The model under review builds one solid part; all positions refer to its coordinate system, in mm. A direction names the side the tool comes from. Coordinates: 2 decimals unless noted, no trailing zeros. Loops run counter-clockwise (first coordinate to the right, second up) from the corner with the lowest first, then second, coordinate; pieces in that order, holes last. Notation, with made-up numbers: M 39.5,82.25 L 69.5,82.25 A9 cw 69.5,94.25 Z; hole C 11,6.5 d8. An arc over 180 degrees is marked long. Use one line per item in the form item = value.
```python
from build123d import *

# Parameters (mm, degrees)
F0_W     = 30
F0_H     = 40
F0_W_2   = 20
F0_H_2   = 8
F2_DEPTH = 3
F1_W     = 20
F1_H     = 3
F3_DEPTH = 1
F4_R     = 0.5


with BuildPart() as f2:
    # F0 (on Top) → F2 (new body)
    with BuildSketch(Plane.XY):
        Rectangle(F0_W, F0_H)
        with Locations((0, 11.941392)):
            Rectangle(F0_W_2, F0_H_2, mode=Mode.SUBTRACT)
    extrude(amount=F2_DEPTH)

    # F1 (on face) → F3 (join)
    with BuildSketch(Plane.XY):
        with Locations((0, 15.365714)):
            Rectangle(F1_W, F1_H)
    extrude(amount=F3_DEPTH)

    # F4
    f4_edges = [f2.edges().sort_by_distance(p)[0] for p in [
        (15, 0, 0),
        (0, 20, 0),
        (-15, 0, 0),
        (0, -20, 0),
        (-15, -20, 1.5),
        (15, -20, 1.5),
        (-15, 20, 1.5),
        (15, 20, 1.5),
    ]]
    fillet(f4_edges, radius=F4_R)


solid = f2.part
```
1. Wall thickness on line 1 along X through (y, z) = (11, 0.65); line 2 along Y through (x, z) = (2.5, 2.5); line 3 along Y through (x, z) = (-3, 0.95): over which ranges is each line inside the solid? List them lowest first. Write a range as from..to.
Response values:
line_1 = -15..-10, 10..15
line_2 = -20..7.94, 15.94..20
line_3 = -20..7.94, 13.87..20
2. Insertion check: P1, Ø8, axis at x = 1.5, y = 9, coming from the -Z side; P2, Ø0.6, axis at x = -4.5, y = 15, coming from the +Z side. Each pin has a flat end and moves straight along its axis. Give the tip position at first contact, or say it passes through.
Response values:
P1 = 0
P2 = 1
3. Add section C-C (y = 13). State the section outline as (x, z) points.
Response values:
outline = M -15,0.5 A0.5 ccw -14.5,0 L -10,0 L -10,3 L -15,3 Z; M 10,0 L 14.5,0 A0.5 ccw 15,0.5 L 15,3 L 10,3 Z
4. Add section B-B (z = 2.05). State the section outline as (x, y) points.
Response values:
outline = M -15,-19.5 A0.5 ccw -14.5,-20 L 14.5,-20 A0.5 ccw 15,-19.5 L 15,19.5 A0.5 ccw 14.5,20 L -14.5,20 A0.5 ccw -15,19.5 Z; hole M -10,7.94 L 10,7.94 L 10,15.94 L -10,15.94 Z
5. The part is to be moulded in two halves that separate along Y. For faces 4 (the face through (-15, 0, 2)), 5 (the face through (-0.1, 13.866, 0.5)), 6 (the face through (0, -20, 2)), say which applies: pulls with the +Y half, pulls with the -Y half, needs draft (parallel to the pull), parting line crosses it, or undercut.
Response values:
face_4 = needs draft
face_5 = undercut
face_6 = pulls with the -Y half
6. Machinability: for faces 1 (the face through (0, 20, 2)), 2 (the face through (0, 7.941, 1)), 3 (the face through (-10, 12, 1)), which of the approach directions +Z, -Z, +X, -X, +Y, -Y give a long, thin tool a straight path to every point of the face, cutting with its end or side? Answer none if there is none.
Response values:
face_1 = +Z, -Z, +X, -X, +Y
face_2 = +Z, -Z
face_3 = +Z
7. Add section A-A (x = -0.5). State the section outline as (y, z) points.
Response values:
outline = M -20,0.5 A0.5 ccw -19.5,0 L 7.94,0 L 7.94,3 L -20,3 Z; M 13.87,0 L 19.5,0 A0.5 ccw 20,0.5 L 20,3 L 15.94,3 L 15.94,1 L 13.87,1 Z
